```python
from build123d import *

# Parameters (mm, degrees)
F1_DEPTH = 10
F2_R     = 0.4
F3_ANGLE = 90


with BuildPart() as f1:
    # F0 (on Front) → F1 (new body)
    with BuildSketch(Plane.XZ):
        Polygon((15.15625, 2.75), (15.15625, 6.758929), (0, 6.758929), (-15.067572, 6.758929), (-15.067572, 2.75), (-13.567572, 2.75), (-13.567572, 5.25), (-9.567572, 5.25), (-9.567572, 0.75), (-12.067572, 0.75), (-12.067572, 0), (-12.067572, -0.75), (-9.567572, -0.75), (-9.567572, -5.25), (-13.567572, -5.25), (-13.567572, -2.75), (-15.067572, -2.75), (-15.067572, -6.758929), (0, -6.758929), (15.15625, -6.758929), (15.15625, -2.75), (13.65625, -2.75), (13.65625, -5.25), (9.65625, -5.25), (9.65625, -0.75), (12.15625, -0.75), (12.15625, 0), (12.15625, 0.75), (9.65625, 0.75), (9.65625, 5.25), (13.65625, 5.25), (13.65625, 2.75), align=None)
    extrude(amount=F1_DEPTH)

    # F2
    f2_edges = [f1.edges().sort_by_distance(p)[0] for p in [
        (15.15625, -5, 2.75),
        (13.65625, -5, 2.75),
        (12.15625, -5, 0.75),
        (12.15625, -5, -0.75),
        (15.15625, -5, -2.75),
        (13.65625, -5, -2.75),
        (-13.567572, -5, -2.75),
        (-15.067572, -5, -2.75),
        (-12.067572, -5, 0.75),
        (-12.067572, -5, -0.75),
        (-13.567572, -5, 2.75),
        (-15.067572, -5, 2.75),
    ]]
    fillet(f2_edges, radius=F2_R)


with BuildPart() as f1_1:
    # F3: moved
    add(f1.part.rotate(Axis((0.044339, -10, -6.758929), (1, 0, 0)), F3_ANGLE))


solid = f1_1.part
```
Geometry check sheet. Reference: the model listing, model coordinates, mm. A direction names the side the tool comes from. Round coordinates to 2 decimals unless told otherwise and drop trailing zeros. Loops run counter-clockwise (first coordinate to the right, second up) from the corner with the lowest first, then second, coordinate; pieces in that order, holes last. Notation, with made-up numbers: (34.5, 79) -> (48.5, 79) arc R26 ccw to (48.5, 118) -> close; hole circle Ø8 at (-38, -27.75). An arc over 180 degrees is marked (long way). Use a Markdown table: item, result.
(1) Mould release check, pull along X, two halves, no side actions. Record for faces 1 (the flat face through (12, -11.509, -2)), 2 (the flat face through (15.156, -22, -2)), 3 (the flat face through (11, -17.509, -2)): released by +X, released by -X, zero draft, split by the parting line, or undercut.
Calculated:
| item | result |
|---|---|
| face 1 | undercut |
| face 2 | released by +X |
| face 3 | zero draft |
(2) Sectioned sample at C-C (y = -15.5). Enter the section's corners in (x, z), then the cut area to 3 significant figures.
Calculated:
| item | result |
|---|---|
| outline | (-9.57, -6.76) -> (9.66, -6.76) -> (9.66, 3.24) -> (-9.57, 3.24) -> close |
| area | 192 mm² |
(3) Scan lines: probe 1 along X at (y, z) = (-20.5, -1.25); probe 2 along Y at (x, z) = (10, 0.25); probe 3 along Y at (x, z) = (13, 2.5). Record each from-to range of solid material in increasing order.
Calculated:
| item | result |
|---|---|
| probe 1 | -15.07 to -13.57, -9.57 to 9.66, 13.66 to 15.16 |
| probe 2 | -23.52 to -22.01, -17.51 to -16.01, -11.51 to -10 |
| probe 3 | -23.52 to -22.01, -11.51 to -10 |
(4) Set-up check for faces 4 (the flat face through (-13.568, -21, -2)), 5 (the flat face through (-11, -16.009, -2)), 6 (the flat face through (0, -23.518, -2)): record each of +Z, -Z, +X, -X, +Y, -Y from which the full face is reachable in a straight line by a thin tool's end or side.
Calculated:
| item | result |
|---|---|
| face 4 | +Z, -Z |
| face 5 | +Z, -Z, -X |
| face 6 | +Z, -Z, +X, -X, -Y |
(5) Sectioned sample at B-B (x = -12.5). Enter the section's corners in (y, z), then the cut area to 3 significant figures.
Calculated:
| item | result |
|---|---|
| outline | (-23.52, -6.76) -> (-22.01, -6.76) -> (-22.01, 3.24) -> (-23.52, 3.24) -> close; (-11.51, -6.76) -> (-10, -6.76) -> (-10, 3.24) -> (-11.51, 3.24) -> close |
| area | 30.2 mm² |
(6) Go/stop test with a flat-tipped pin: P1, Ø1.5, axis at y = -17, z = -4, coming from the -X side. Record where the tip stops, or that it passes through.
Calculated:
| item | result |
|---|---|
| P1 | x = -12.07 |
(7) Sectioned sample at A-A (y = -20.25). Enter the section's corners in (x, z), then the cut area to 3 significant figures.
Calculated:
| item | result |
|---|---|
| outline | (-15.07, -6.76) -> (-13.57, -6.76) -> (-13.57, 3.24) -> (-15.07, 3.24) -> close; (-9.57, -6.76) -> (9.66, -6.76) -> (9.66, 3.24) -> (-9.57, 3.24) -> close; (13.66, -6.76) -> (15.16, -6.76) -> (15.16, 3.24) -> (13.66, 3.24) -> close |
| area | 222 mm² |
